Work out the finished part from the listing and answer in its coordinate system (mm). A direction names the side the tool comes from. Round coordinates to 2 decimals unless told otherwise and drop trailing zeros. Write each loop counter-clockwise with the first axis right and the second up, starting at its lowest first coordinate (ties: lowest second). Pieces come first, ordered by that corner, then holes. Notation, with made-up numbers: M 74,-27 L 89,-27 A18 ccw 89,-21 Z; hole C 56.25,-37 d6. An arc over 180 degrees is marked long. One line per item, written item: value. Start each with the question number.
Q1. Given pin 1 Ø1 at (x, y) = (-2.5, 1) entering from -Z; pin 2 Ø14 at (x, z) = (-2.5, -13.5) entering from +Y; pin 3 Ø3 at (x, y) = (6, 2.5) entering from +Z; pin 4 Ø3 at (x, z) = (-8.5, -19.5) entering from -Y, each flat-ended and moving along its own axis, determine where each tip first touches the part or whether it passes through.
Q2. Find section D-D (y = 4.3). Write down the section's boundary in (x, z), and give its area (3 significant figures).
Q3. Find section C-C (x = -7.25). Write down the section's boundary in (y, z).
Q4. Find section B-B (z = -3.25). Write down the section's boundary in (x, y), and give its area (3 significant figures).
Q5. A tool of negligible diameter and unlimited length cuts with its end or side. For faces 1 (the cylindrical face through (-4.16, 3.98, -26.14)), 2 (the flat face through (-13.81, 1.01, -12.01)), from which of +Z, -Z, +X, -X, +Y, -Y can it reach the whole face along a straight path? Write none if from no direction.
Q6. The mould has two halves that part along Z. Classify faces 3 (the cylindrical face through (-6.79, 0.99, -3.42)), 4 (the flat face through (-4, 6, -25)), 5 (the cylindrical face through (10.401, 1.014, -21.298)): released by +Z, released by -Z, zero draft, split by the parting line, or undercut.
Q7. Consider probe 1 along Y at (x, z) = (-9.5, -21); probe 2 along X at (y, z) = (0.55, -9); probe 3 along X at (y, z) = (0.55, -13). Determine where each line is inside the solid, lowest interval first.
from build123d import *

# Parameters (mm, degrees)
BOSS_EXTRUDE1_DEPTH = 2
FILLET1_R           = 2.5
SKETCH2_R           = 1.5
SKETCH2_R_2         = 1.75
CUT_EXTRUDE1_DEPTH  = 2
CUT_EXTRUDE2_REACH  = 34.399
BOSS_EXTRUDE2_START = -2
SKETCH6_R           = 1.5
BOSS_EXTRUDE2_DEPTH = 2
BOSS_EXTRUDE3_START = -2
BOSS_EXTRUDE3_DEPTH = 2
FILLET2_START       = -1
FILLET2_DEPTH       = 4
FILLET2_2_DEPTH     = 2
CUT_EXTRUDE3_DEPTH  = 2
FILLET3_R           = 4
SKETCH11_R          = 1.5
BOSS_EXTRUDE4_DEPTH = 4
FILLET6_R           = 0.25


with BuildPart() as part:
    # Sketch1 → Boss-Extrude1 (new body)
    with BuildSketch(Plane(origin=(0, 0, 0), x_dir=(1, 0, 0), z_dir=(0, 1, 0))):
        with BuildLine():
            ThreePointArc((15.125, 22.967027997), (-1.263298306, 27.470967901), (-17.169059596, 21.48193177))
            ThreePointArc((-17.169059596, 21.48193177), (-11.803604023, 8.168176911), (0, 0))
            ThreePointArc((0, 0), (4.120883639, 13.75), (15.125, 22.967027997))
        make_face()
    extrude(amount=BOSS_EXTRUDE1_DEPTH)

    # Fillet1
    fillet1_edges = [part.edges().sort_by_distance(p)[0] for p in [
        (-17.169059596, 1, -21.48193177),
        (15.125, 1, -22.967027997),
    ]]
    fillet(fillet1_edges, radius=FILLET1_R)

    # Sketch2 → Cut-Extrude1 (cut)
    with BuildSketch(Plane(origin=(0, 2, 0), x_dir=(1, 0, 0), z_dir=(0, 1, 0))):
        with Locations(Location((-4.226868107, 24.640080885, 0), (0, 0, 270))):
            Circle(SKETCH2_R)
        with Locations(Location((9.875, 22.967027997, 0), (0, 0, 270))):
            Circle(SKETCH2_R_2)
    extrude(amount=-CUT_EXTRUDE1_DEPTH, mode=Mode.SUBTRACT)

    # Sketch3 → Cut-Extrude2 (cut, up to next)
    with BuildSketch(Plane(origin=(0, 2, 0), x_dir=(1, 0, 0), z_dir=(0, 1, 0)), mode=Mode.PRIVATE) as cut_extrude2_sk1:
        with BuildLine():
            Line((-15.980917027, 15.838569726), (-12.020745702, 24.733614228))
            ThreePointArc((-12.020745702, 24.733614228), (-14.04148027, 23.645017061), (-15.964394934, 22.391696997))
            ThreePointArc((-15.964394934, 22.391696997), (-16.816313344, 21.328273965), (-16.984031989, 19.976052098))
            ThreePointArc((-16.984031989, 19.976052098), (-16.570708205, 17.885919028), (-15.980917027, 15.838569726))
        make_face()
    cut_extrude2_tool1 = extrude(cut_extrude2_sk1.sketch, amount=-CUT_EXTRUDE2_REACH, mode=Mode.PRIVATE) & part.part
    add(cut_extrude2_tool1.solids().sort_by_distance((-15.061244, 2, -20.693622))[0], mode=Mode.SUBTRACT)

    # Sketch6 → Boss-Extrude2 (add)
    with BuildSketch(Plane.XZ.offset(BOSS_EXTRUDE2_START)):
        with Locations((-4.226868107, -24.640080885)):
            Circle(SKETCH6_R)
    extrude(amount=BOSS_EXTRUDE2_DEPTH)

    # Sketch7 → Boss-Extrude3 (add)
    with BuildSketch(Plane(origin=(0, 2, 0), x_dir=(1, 0, 0), z_dir=(0, 1, 0)).offset(BOSS_EXTRUDE3_START)):
        with BuildLine():
            Line((9.313984882, 19.466610638), (11.248778971, 20.27693074))
            ThreePointArc((11.248778971, 20.27693074), (11.386576571, 20.3697006), (11.525, 20.461534033))
            ThreePointArc((11.525, 20.461534033), (12.863352389, 23.23113025), (11.06, 25.723071356))
            ThreePointArc((11.06, 25.723071356), (10.846265511, 25.813921137), (10.631784841, 25.902995022))
            Line((10.631784841, 25.902995022), (8.903638019, 26.018747665))
            ThreePointArc((8.903638019, 26.018747665), (9.890276319, 25.659938315), (10.8625, 25.263730796))
            ThreePointArc((10.8625, 25.263730796), (12.365293657, 23.187113207), (11.25, 20.879116361))
            ThreePointArc((11.25, 20.879116361), (10.26505719, 20.196075371), (9.313984882, 19.466610638))
        make_face()
    extrude(amount=BOSS_EXTRUDE3_DEPTH)

    # Fillet2: read off the stored shape, not the designer's step
    # Fillet2 outline → Fillet2 (cut)
    with BuildSketch(Plane(origin=(0, 0, 0), x_dir=(1, 0, 0), z_dir=(0, 1, 0)).offset(FILLET2_START)):
        with BuildLine():
            ThreePointArc((11.525, 20.461534033), (11.178047435, 20.264564275), (10.816495082, 20.095883915))
            Line((10.816495082, 20.095883915), (11.248778971, 20.27693074))
            ThreePointArc((11.248778971, 20.27693074), (11.386576571, 20.3697006), (11.525, 20.461534033))
        make_face()
        with BuildLine():
            Line((10.631784841, 25.902995022), (9.853687309, 25.955112611))
            ThreePointArc((9.853687309, 25.955112611), (10.463996888, 25.876279494), (11.06, 25.723071356))
            ThreePointArc((11.06, 25.723071356), (10.846265511, 25.813921137), (10.631784841, 25.902995022))
        make_face()
    extrude(amount=FILLET2_DEPTH, mode=Mode.SUBTRACT)

    # Fillet2 2 outline → Fillet2 2 (add)
    with BuildSketch(Plane(origin=(0, 0, 0), x_dir=(1, 0, 0), z_dir=(0, 1, 0))):
        with BuildLine():
            ThreePointArc((9.313984882, 19.466610638), (8.990075455, 19.201101949), (8.670659365, 18.930204289))
            ThreePointArc((8.670659365, 18.930204289), (9.30523679, 19.395787738), (10.005013016, 19.756023341))
            Line((10.005013016, 19.756023341), (9.313984882, 19.466610638))
        make_face()
        with BuildLine():
            Line((8.903638019, 26.018747665), (9.535077314, 25.97645336))
            ThreePointArc((9.535077314, 25.97645336), (8.936180246, 26.053104962), (8.350889065, 26.201386448))
            ThreePointArc((8.350889065, 26.201386448), (8.627746835, 26.111529725), (8.903638019, 26.018747665))
        make_face()
    extrude(amount=FILLET2_2_DEPTH)

    # Sketch8 → Cut-Extrude3 (cut)
    with BuildSketch(Plane(origin=(0, 2, 0), x_dir=(1, 0, 0), z_dir=(0, 1, 0))):
        Polygon((-17.225521171, 19.396093794), (-10.650323335, 5.173654997), (-21.381773126, 15.240189751), align=None)
    extrude(amount=-CUT_EXTRUDE3_DEPTH, mode=Mode.SUBTRACT)

    # Fillet3
    fillet3_edges = [part.edges().sort_by_distance(p)[0] for p in [
        (-15.784646242, 1, -16.279418676),
        (-12.383702581, 1, -8.923029671),
    ]]
    fillet(fillet3_edges, radius=FILLET3_R)

    # Sketch11 → Boss-Extrude4 (add)
    with BuildSketch(Plane(origin=(0, 2, 0), x_dir=(1, 0, 0), z_dir=(0, 1, 0))):
        with Locations(Location((-4.226868107, 24.640080885, 0), (0, 0, 270))):
            Circle(SKETCH11_R)
    extrude(amount=BOSS_EXTRUDE4_DEPTH)

    # Fillet6
    fillet6_edges = [part.edges().sort_by_distance(p)[0] for p in [
        (-4.226868107, 2, -26.140080885),
        (-4.226868107, 6, -26.140080885),
    ]]
    fillet(fillet6_edges, radius=FILLET6_R)


solid = part.part
The answers:
1. pin 1: z = -27.43
1. pin 2: y = 2
1. pin 3: z = -14.43
1. pin 4: y = 0
2. outline: C -4.23,-24.64 d3
2. area: 7.07 mm2
3. outline: M 0,-26.53 L 2,-26.53 L 2,-3.76 L 0,-3.76 Z
4. outline: M -6.55,0 L 0.21,0 L 0.21,2 L -6.55,2 Z
4. area: 13.5 mm2
5. face 1: +Y
5. face 2: +Z, -X, +Y, -Y
6. face 3: released by +Z
6. face 4: zero draft
6. face 5: undercut
7. probe 1: 0 to 2
7. probe 2: -12.4 to 1.68
7. probe 3: -14.27 to 3.65
